Check sheet for the drawn part. Datum: minimum x, y, z corner. Units: mm. A direction names the side the tool comes from. Coordinates: 2 decimals unless noted, no trailing zeros. Loops run counter-clockwise (first coordinate to the right, second up) from the corner with the lowest first, then second, coordinate; pieces in that order, holes last. Notation, with made-up numbers: (33.25, 29.5) - (63.25, 29.5) arc R11 ccw to (63.25, 38.5) - close; hole circle Ø1 at (47.25, -25). An arc over 180 degrees is marked (long way). Answer as CSV lines item,"result". Start each with the question number.
1. Cross-section at D-D (z = 10). Enter the section's corners in (x, y).
2. Cross-section at B-B (z = 17.5). Enter the section's corners in (x, y), plus the area to 3 significant figures.
3. Gauge pin test, flat ends, axial feed: P1, Ø4, axis at x = 26.5, y = 8, coming from the -Z side; P2, Ø3, axis at y = 4, z = 16.5, coming from the +X side; P3, Ø1.5, axis at y = 9, z = 2, coming from the -X side; P4, Ø5, axis at x = 4, y = 6.5, coming from the +Z side. Record the tip position at first contact, or that the pin passes through.
4. Release check for a two-part mould opening along X. For the marked faces 1, 2, 3 and 4 record: pulls with the +X half, pulls with the -X half, needs draft (parallel to the pull), parting line crosses it, or undercut.
5. Material ranges on line 1 (Z direction, x = 6, y = 5); line 2 (X direction, y = 4.25, z = 10.25); line 3 (X direction, y = 0.5, z = 14), recorded low to high. Write a range as [from, to].
6. Cross-section at A-A (x = 5). Enter the section's corners in (y, z), plus the area to 3 significant figures.
7. Set-up check for the marked faces 5 and 6: record each of +Z, -Z, +X, -X, +Y, -Y from which the full face is reachable in a straight line by a thin tool's end or side.
8. Cross-section at C-C (y = 5). Enter the section's corners in (x, z), plus the area to 3 significant figures.
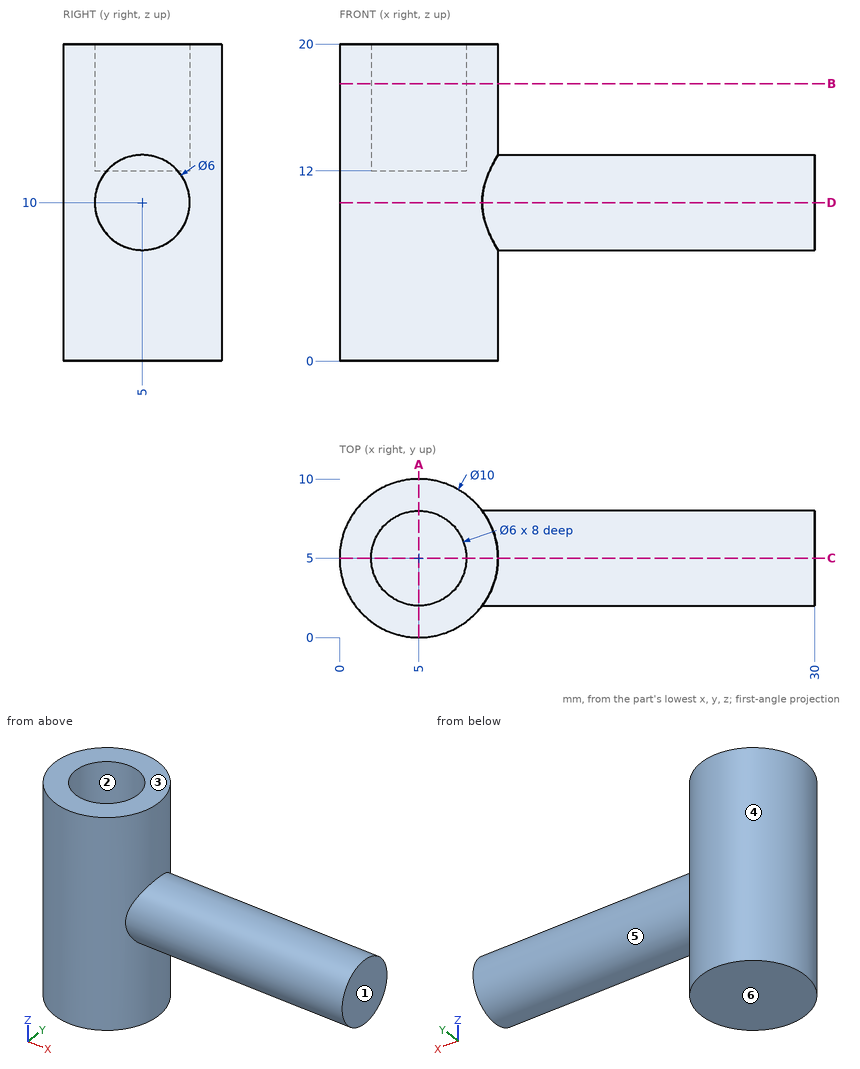
Values follow:
1,outline,"(9, 2) - (30, 2) - (30, 8) - (9, 8) arc R5 ccw (long way) to start"
2,outline,"circle Ø10 at (5, 5); hole circle Ø6 at (5, 5)"
2,area,"50.3 mm²"
3,P1,"stops at z = 7.17"
3,P2,"stops at x = 10"
3,P3,"stops at x = 1.2"
3,P4,"stops at z = 20"
4,face 1,"pulls with the +X half"
4,face 2,"undercut"
4,face 3,"needs draft"
4,face 4,"parting line crosses it"
5,line 1,"z = [0, 12]"
5,line 2,"x = [0.06, 30]"
5,line 3,"x = [2.82, 7.18]"
6,outline,"(0, 0) - (10, 0) - (10, 20) - (8, 20) - (8, 12) - (2, 12) - (2, 20) - (0, 20) - close"
6,area,"152 mm²"
7,face 5,"+X"
7,face 6,"-Z, +X, -X, +Y, -Y"
8,outline,"(0, 0) - (10, 0) - (10, 7) - (30, 7) - (30, 13) - (10, 13) - (10, 20) - (8, 20) - (8, 12) - (2, 12) - (2, 20) - (0, 20) - close"
8,area,"272 mm²"
